For this review, take the finished solid that the model builds, in its own axes (mm). Coordinates: 2 decimals unless noted, no trailing zeros. Order: outer loops, then holes, each group sorted by start corner. A loop starts at its lowest first (then second) coordinate and runs counter-clockwise, first axis right, second up. Notation, with made-up numbers: M -37.75,28 L -19.75,28 A27 cw -19.75,66 Z; hole C 46.25,54.25 d3. An arc over 180 degrees is marked long. Use CSV: the item, a comma, the result in double quotes.
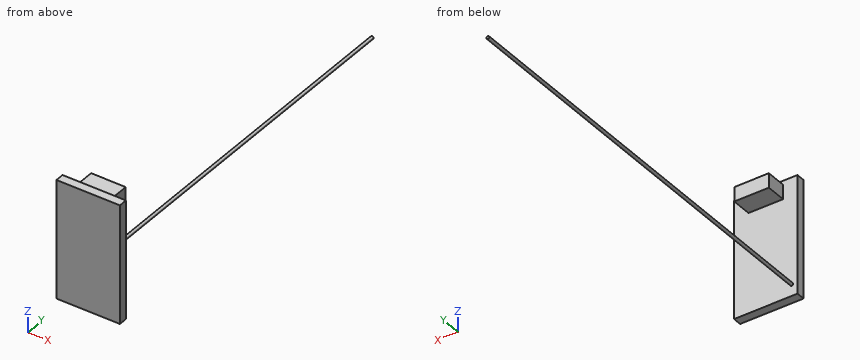
Autodesk Fusion 360 part; units mm, degrees
sketch "Sketch1" plane through (0, 0, 0) normal (0, 1, 0) x (1, 0, 0)
  line L0 (0, 0) -> (22, 0)
  line L1 (22, 0) -> (22, -41)
  line L2 (22, -41) -> (0, -41)
  line L3 (0, -41) -> (0, 0)
  dimension "d1" = 22
  dimension "d2" = 41
extrude "Extrude1" add sketch "Sketch1" along normal blind 3
sketch "Sketch2" plane through (0, 3, 0) normal (0, 1, 0) x (-1, 0, 0)
  line L0 (0, 41) -> (-22, 41)
  line L1 (-22, 41) -> (-22, 0)
  line L2 (-22, 0) -> (0, 0)
  line L3 (0, 0) -> (0, 41)
  line L4 (-5, 34.6463) -> (-17, 34.6463)
  line L5 (-17, 34.6463) -> (-17, 39.6463)
  line L6 (-17, 39.6463) -> (-5, 39.6463)
  line L7 (-5, 39.6463) -> (-5, 34.6463)
  dimension "d5" = 12
  dimension "d6" = 5
  dimension "d7" = 5
  dimension "d8" = 5
extrude "Extrude2" add sketch "Sketch2" along normal blind 7 contours L4 L5 L6 L7
sketch "Sketch3" plane through (0, 3, 0) normal (0, 1, 0) x (-1, 0, 0)
  line L0 (-5, 39.6463) -> (-5, 34.6463)
  line L1 (-5, 34.6463) -> (-17, 34.6463)
  line L2 (-17, 34.6463) -> (-17, 39.6463)
  line L3 (-17, 39.6463) -> (-5, 39.6463)
  line L4 (0, 41) -> (-22, 41)
  line L5 (-22, 41) -> (-22, 0)
  line L6 (-22, 0) -> (0, 0)
  line L7 (0, 0) -> (0, 41)
  circle A0 centre (-2, 4) radius 0.5
  dimension "d11" = 1
extrude "Extrude3" add sketch "Sketch3" along normal blind 150 contours A0
Item 1: Clearance check with flat-ended pins moving along their axes: pin 1 Ø5.5 at (x, y) = (12.5, 6) entering from -Z; pin 2 Ø8 at (x, z) = (10, 24) entering from -Y; pin 3 Ø5.5 at (y, z) = (8, 37.5) entering from +X; pin 4 Ø5.5 at (x, z) = (10, 36) entering from +Y. State where each tip first meets the part, or that it passes through.
Solutions:
pin 1,"z = 34.65"
pin 2,"y = 0"
pin 3,"x = 17"
pin 4,"y = 10"
Item 2: Add section A-A on x = 13.5. State the section outline as (y, z) points.
Solutions:
outline,"M 0,0 L 3,0 L 3,34.65 L 10,34.65 L 10,39.65 L 3,39.65 L 3,41 L 0,41 Z"
Item 3: Add section B-B on y = 114.5. State the section outline as (x, z) points, and give its area (3 significant figures).
Solutions:
outline,"C 2,4 d1"
area,"0.785 mm^2"
Item 4: To check wall thickness, follow line 1 along Y through (x, z) = (6.75, 31); line 2 along Y through (x, z) = (5.5, 38.5). State the ranges of each line that lie inside material, in increasing order. Write a range as [from, to].
Solutions:
line 1,"[0, 3]"
line 2,"[0, 10]"
Item 5: Add section C-C on z = 23. State the section outline as (x, y) points.
Solutions:
outline,"M 0,0 L 22,0 L 22,3 L 0,3 Z"
